The model under review builds one solid part; all positions refer to its coordinate system, in mm. A direction names the side the tool comes from. Coordinates: 2 decimals unless noted, no trailing zeros. Write each loop counter-clockwise with the first axis right and the second up, starting at its lowest first coordinate (ties: lowest second). Pieces come first, ordered by that corner, then holes. Notation, with made-up numbers: (39, 78.25) - (94, 78.25) arc R21 cw to (94, 113.25) - close; hole circle Ø1 at (70, 59.25). An arc over 180 degrees is marked (long way). Put each result on its own line as item: value.
from build123d import *

# Parameters (mm, degrees)
F1_DEPTH = 60
F3_DEPTH = 25
F5_DEPTH = 25


with BuildPart() as f1:
    # F0 (on Front) → F1 (new body, symmetric)
    with BuildSketch(Plane.XZ):
        Polygon((-120, 148.1876587842), (0, 0), (350, 0), (500, 54.5955351399), (491.4494964169, 78.0878506596), (345.5918254823, 25), (11.9243883175, 25), (-100.5713509636, 163.9206685605), align=None)
    extrude(amount=F1_DEPTH, both=True)

    # F2 (on face) → F3 (cut)
    with BuildSketch(Plane(origin=(19.4286490364, 0, 15.7330097762), x_dir=(0, 1, 0), z_dir=(0.7771459615, 0, 0.629320391))):
        Polygon((-60, 190.6818874879), (-60, 11.9243883175), (-34.7125157714, 190.6818874879), align=None)
        Polygon((34.7125157714, 190.6818874879), (60, 11.9243883175), (60, 190.6818874879), align=None)
    extrude(amount=-F3_DEPTH, mode=Mode.SUBTRACT)

    # F4 (on face) → F5 (cut)
    with BuildSketch(Plane(origin=(32.391718871, 0, -88.9955161755), x_dir=(0.9396926208, 0, 0.3420201433), z_dir=(-0.3420201433, 0, 0.9396926208))):
        Polygon((488.5190831465, 60), (333.3005917928, 60), (488.5190831465, 40), align=None)
        Polygon((358.5190831465, -20), (488.5190831465, -20), (488.5190831465, 20), (358.5190831465, 20), (358.5190831465, 0), align=None)
        Polygon((488.5190831465, -40), (333.3005917928, -60), (488.5190831465, -60), align=None)
    extrude(amount=-F5_DEPTH, mode=Mode.SUBTRACT)


solid = f1.part
1. For pin 1 Ø3 at (x, z) = (-33.5, 64) entering from -Y; pin 2 Ø2 at (y, z) = (-3, 55.5) entering from +X; pin 3 Ø6 at (x, y) = (192.5, 12) entering from +Z, all flat-tipped, find the tip position at first contact; note any pin that passes through.
Determined:
pin 1: stops at y = -51.88
pin 2: stops at x = -11.96
pin 3: stops at z = 25
2. Consider section A-A on y = 5. State the section outline as (x, z) points, plus the area to 3 significant figures.
Determined:
outline: (-120, 148.19) - (0, 0) - (350, 0) - (377.84, 10.13) - (369.29, 33.63) - (345.59, 25) - (11.92, 25) - (-100.57, 163.92) - close
area: 13,800 mm^2
3. Consider section B-B on x = 404. State the section outline as (y, z) points, plus the area to 3 significant figures.
Determined:
outline: (-53.16, 19.65) - (-20, 19.65) - (-20, 46.26) - (-51.99, 46.26) - close; (20, 19.65) - (53.16, 19.65) - (51.99, 46.26) - (20, 46.26) - close
area: 1,730 mm^2
4. The part is to be moulded in two halves that separate along X. For faces 1 (the flat face through (171, 60, 13)), 2 (the flat face through (403.34, 25.83, 46.02)), 3 (the flat face through (407.28, 25.83, 20.85)), say which applies: +X half, -X half, draft (parallel to the pull), parting line (faces both ways), or undercut.
Determined:
face 1: draft
face 2: undercut
face 3: +X half
5. Machinability: for faces 4 (the flat face through (373.505, 0.28, 22.044)), 5 (the flat face through (495.785, 29.86, 66.177)), 6 (the flat face through (181, -1, 25)), which of the approach directions +Z, -Z, +X, -X, +Y, -Y give a long, thin tool a straight path to every point of the face, cutting with its end or side? Answer none if there is none.
Determined:
face 4: +Z, +X
face 5: +Z, +X, +Y, -Y
face 6: +Z, +Y, -Y
6. Consider section C-C on z = 63.5. State the section outline as (x, y) points.
Determined:
outline: (-51.42, -50.13) - (-19.25, -52.99) - (-19.25, 52.99) - (-51.42, 50.13) - close; (451.37, -45.5) - (496.76, -40) - (496.76, -20) - (451.37, -20) - close; (451.37, 20) - (496.76, 20) - (496.76, 40) - (451.37, 45.5) - close
7. To check wall thickness, follow probe 1 along Z at (x, y) = (213, -37); probe 2 along Z at (x, y) = (5, 23); probe 3 along X at (y, z) = (1.5, 38). State the ranges of each line that lie inside material, in increasing order.
Determined:
probe 1: z = 0 to 25
probe 2: z = 0 to 33.55
probe 3: x = -30.77 to 1.4
8. Consider section D-D on z = 40. State the section outline as (x, y) points.
Determined:
outline: (-32.39, -54.41) - (-0.22, -57.27) - (-0.22, 57.27) - (-32.39, 54.41) - close; (386.8, -54.35) - (459.9, -45.5) - (459.9, -20) - (386.8, -20) - close; (386.8, 20) - (459.9, 20) - (459.9, 45.5) - (386.8, 54.35) - close
